Check sheet for the modelled part. Datum: model origin and axes. Units: mm. Face numbers are marked on the shaded views. A direction names the side the tool comes from. Round coordinates to 2 decimals unless told otherwise and drop trailing zeros. Loops run counter-clockwise (first coordinate to the right, second up) from the corner with the lowest first, then second, coordinate; pieces in that order, holes last. Notation, with made-up numbers: (22, 16.25) - (43, 16.25) arc R19 cw to (43, 39.25) - close; hole circle Ø11 at (-22, -20.5). An arc over 180 degrees is marked (long way). Put each result on its own line as item: value. Start each with the question number.
Item 1: Section check A-A, the plane z = -27.5. Record the cut outline in (x, y), and give its area (4 significant figures).
Item 2: Tool access check on the marked faces 1, 2 and 3. Record the directions out of +Z, -Z, +X, -X, +Y, -Y that give a thin tool (end or side, any length) a straight path to the whole face; none if there is none.
Item 3: Gauge pin test, flat ends, axial feed: pin 1 Ø3.5 at (x, z) = (0, -10) entering from +Y; pin 2 Ø2.5 at (x, z) = (0, -45) entering from +Y; pin 3 Ø23 at (y, z) = (32, -27.5) entering from -X. Record the tip position at first contact, or that the pin passes through.
Item 4: Draft check along Z on the marked faces 4 and 5. Enter one of: pulls with the +Z half, pulls with the -Z half, needs draft (parallel to the pull), parting line crosses it, or undercut.
Item 5: Section check D-D, the plane z = -10. Record the cut outline in (x, y).
Item 6: Material ranges on line 1 along Z through (x, y) = (0, 11.05); line 2 along Y through (x, z) = (-5.75, -39), recorded low to high.
Item 7: Section check C-C, the plane x = 0. Record the cut outline in (y, z).
Item 8: Section check B-B, the plane y = 8. Record the cut outline in (x, z), and give its area (3 significant figures).
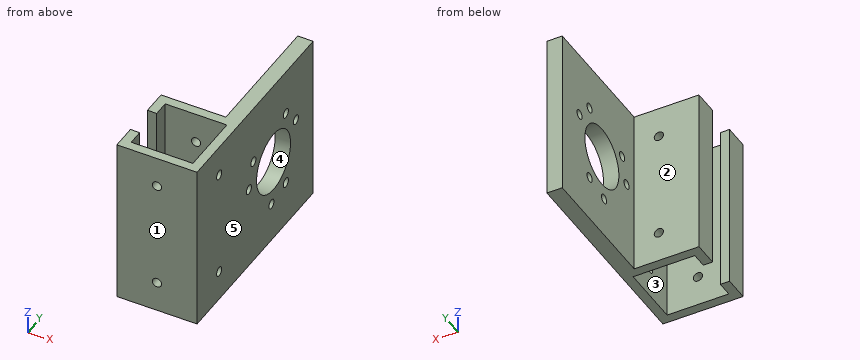
Autodesk Inventor part; units mm, degrees
ref_plane "YZ Plane" through (0, 0, 0) normal (1, 0, 0) x (0, 1, 0)
ref_plane "XZ Plane" through (0, 0, 0) normal (0, 1, 0) x (-1, 0, 0)
ref_plane "XY Plane" through (0, 0, 0) normal (0, 0, 1) x (1, 0, 0)
sketch "Sketch1" plane through (0, 0, 0) normal (0, 0, 1) x (1, 0, 0)
  line L0 (10, 10) -> (-10, 10) construction
  line L1 (-10, 10) -> (-10, -10) construction
  line L2 (-10, -10) -> (10, -10) construction
  line L3 (10, -10) -> (10, 10) construction
  line L4 (-7, -7) -> (-7, 7) construction
  line L5 (-7, 7) -> (7, 7) construction
  line L6 (7, 7) -> (7, -7) construction
  line L7 (7, -7) -> (-7, -7) construction
  line L8 (10, 10) -> (-10, 10)
  line L9 (-10, 10) -> (-10, -10)
  line L10 (-10, -10) -> (10, -10)
  line L11 (10, -10) -> (10, 10)
  line L12 (13, 13) -> (-13, 13)
  line L13 (-13, 13) -> (-13, -13)
  line L14 (-13, -13) -> (13, -13)
  line L15 (13, -13) -> (13, 13)
  point P0 (0, 0)
  dimension "d1" = 3
  dimension "d2" = 3
  dimension "d3" = 3
  dimension "d4" = 3
extrude "Extrusion1" add sketch "Sketch1" against normal blind 55
sketch "Sketch2" plane through (-13, -13, 0) normal (-1, 0, 0) x (0, 0, 1)
  line L0 (-80.4804, 18) -> (40.5, 18)
  line L1 (40.5, 18) -> (40.5, 8)
  line L2 (40.5, 8) -> (-80.4804, 8)
  line L3 (-80.4804, 8) -> (-80.4804, 18)
  line L4 (0, 26) -> (-55, 26)
  point P0 (0, 13)
  dimension "d7" = 10
  dimension "d8" = 8
extrude "Extrusion2" cut sketch "Sketch2" against normal blind 15.3125
sketch "Sketch3" plane through (-13, 13, 0) normal (0, 1, 0) x (1, 0, 0)
  line L0 (26, 0) -> (0, 0)
  line L1 (3, 55) -> (23, 55)
  line L2 (26, 0) -> (21, 0)
  line L3 (21, 0) -> (21, 55)
  line L4 (21, 55) -> (26, 55)
  line L5 (26, 55) -> (26, 0)
  point P0 (13, 0)
  dimension "d11" = 5
extrude "Extrusion3" add sketch "Sketch3" along normal blind 42.3
sketch "Sketch4" plane through (13, -13, 0) normal (1, 0, 0) x (0, 0, -1)
  line L0 (0, 26) -> (55, 26)
  circle A0 centre (27.5, 45) radius 18
  line L1 (0, 68.3) -> (55, 68.3)
  circle A1 centre (27.5, 45) radius 3
  point P0 (0, 13)
  point P1 (27.5, 68.3)
  dimension "d14" = 36
  dimension "d15" = 19
  dimension "d16" = 6
extrude "Extrusion4" cut sketch "Sketch4" against normal blind 42.3 contours A1
sketch "Sketch5" plane through (13, -13, 0) normal (1, 0, 0) x (0, 0, -1)
  circle A0 centre (27.5, 45) radius 3
  circle A1 centre (27.5, 45) radius 10
  point P0 (0, 13)
  dimension "d19" = 20
extrude "Extrusion5" cut sketch "Sketch5" against normal blind 42.3
sketch "Sketch6" plane through (13, -13, 0) normal (1, 0, 0) x (0, 0, -1)
  circle A0 centre (27.5, 30.5) radius 1.5
  circle A1 centre (19.1831, 33.1223) radius 1.495
  circle A2 centre (14.9426, 52.25) radius 1.5
  circle A3 centre (21.372, 58.1415) radius 1.495
  circle A4 centre (40.0574, 52.25) radius 1.5
  circle A5 centre (41.9448, 43.7362) radius 1.495
  point P0 (0, 13)
extrude "Extrusion6" cut sketch "Sketch6" against normal blind 42.3
sketch "Sketch7" plane through (13, -13, 0) normal (1, 0, 0) x (0, 0, -1)
  circle A0 centre (10, 13) radius 1.5
  circle A1 centre (45, 13) radius 1.5
  line L0 (0, 0) -> (0, 68.3)
  line L1 (55, 0) -> (55, 68.3)
  point P0 (0, 13)
  dimension "d24" = 3
  dimension "d25" = 3
  dimension "d26" = 10
  dimension "d27" = 10
extrude "Extrusion7" cut sketch "Sketch7" against normal blind 10
sketch "Sketch8" plane through (-13, -13, 0) normal (0, -1, 0) x (1, 0, 0)
  circle A0 centre (13, -10) radius 1.5
  circle A1 centre (13, -45) radius 1.5
  line L0 (26, -55) -> (0, -55)
  line L1 (0, 0) -> (26, 0)
  point P0 (13, 0)
  point P1 (13, 0)
  point P2 (13, 0)
  dimension "d30" = 3
  dimension "d31" = 3
  dimension "d32" = 10
  dimension "d33" = 10
extrude "Extrusion8" cut sketch "Sketch8" against normal through all
properties part number "enc holder"
Check result:
1. outline: (-13, -13) - (13, -13) - (13, 16) - (8, 16) - (8, 13) - (-13, 13) - (-13, 5) - (-10, 5) - (-10, 10) - (10, 10) - (10, -10) - (-10, -10) - (-10, -5) - (-13, -5) - close; (8, 19) - (13, 19) - (13, 22) - (8, 22) - close; (8, 42) - (13, 42) - (13, 55.3) - (8, 55.3) - close
1. area: 342.5 mm²
2. face 1: +Z, -Z, +X, -X, -Y
2. face 2: +Z, -Z, -X, +Y
2. face 3: +Z, -Z
3. pin 1: y = 13
3. pin 2: through
3. pin 3: x = 8
4. face 4: undercut
4. face 5: needs draft
5. outline: (-13, -13) - (-1.5, -13) - (-1.5, -10) - (-10, -10) - (-10, -5) - (-13, -5) - close; (-13, 5) - (-10, 5) - (-10, 10) - (-1.5, 10) - (-1.5, 13) - (-13, 13) - close; (1.5, -13) - (13, -13) - (13, -1.5) - (10, -1.5) - (10, -10) - (1.5, -10) - close; (1.5, 10) - (10, 10) - (10, 1.5) - (13, 1.5) - (13, 55.3) - (8, 55.3) - (8, 13) - (1.5, 13) - close
6. line 1: -55 to -46.5, -43.5 to -11.5, -8.5 to 0
6. line 2: -13 to -10, 10 to 13
7. outline: (-13, -55) - (-10, -55) - (-10, -46.5) - (-13, -46.5) - close; (-13, -43.5) - (-10, -43.5) - (-10, -11.5) - (-13, -11.5) - close; (-13, -8.5) - (-10, -8.5) - (-10, 0) - (-13, 0) - close; (10, -55) - (13, -55) - (13, -46.5) - (10, -46.5) - close; (10, -43.5) - (13, -43.5) - (13, -11.5) - (10, -11.5) - close; (10, -8.5) - (13, -8.5) - (13, 0) - (10, 0) - close
8. outline: (-13, -55) - (-10, -55) - (-10, 0) - (-13, 0) - close; (10, -55) - (13, -55) - (13, 0) - (10, 0) - close
8. area: 330 mm²
